from build123d import *

# Parameters (mm, degrees)
EXTRUDE1_DEPTH                         = 10
F_4_0_4_DIAMETER_HOLE1_D               = 3.9
F_4_0_4_DIAMETER_HOLE1_DEPTH           = 15
F_4_0_4_DIAMETER_HOLE1_ON_FACE_2_D     = 3.9
F_4_0_4_DIAMETER_HOLE1_ON_FACE_2_DEPTH = 15
SKETCH3_W                              = 10
SKETCH3_H                              = 8
EXTRUDE2_DEPTH                         = 10
F_4_0_4_DIAMETER_HOLE2_D               = 3.9
F_4_0_4_DIAMETER_HOLE2_DEPTH           = 15


with BuildPart() as part:
    # Sketch1 → Extrude1 (new body)
    with BuildSketch(Plane.XY):
        Polygon((-43.75, -15), (-43.75, -5), (23.75, 15), (43.75, 15), (43.75, -15), align=None)
    extrude(amount=EXTRUDE1_DEPTH)

    # Ø4.0 (4) Diameter Hole1
    with Locations(Plane(origin=(-43.75, -10, 5), x_dir=(0, 0, -1), z_dir=(-1, 0, 0))):
        with Locations((0, 0)):
            Hole(F_4_0_4_DIAMETER_HOLE1_D / 2, depth=F_4_0_4_DIAMETER_HOLE1_DEPTH)

    # Ø4.0 (4) Diameter Hole1 on face 2
    with Locations(Plane(origin=(43.75, -10, 5), x_dir=(0, 0, 1), z_dir=(1, 0, 0))):
        with Locations((0, 0), (0, -20)):
            Hole(F_4_0_4_DIAMETER_HOLE1_ON_FACE_2_D / 2, depth=F_4_0_4_DIAMETER_HOLE1_ON_FACE_2_DEPTH)

    # Sketch3 → Extrude2 (add)
    with BuildSketch(Plane.XY):
        with Locations((-38.75, -19)):
            Rectangle(SKETCH3_W, SKETCH3_H)
    extrude(amount=EXTRUDE2_DEPTH)

    # Ø4.0 (4) Diameter Hole2
    with Locations(Plane(origin=(-43.75, -18, 5), x_dir=(0, 0, -1), z_dir=(-1, 0, 0))):
        with Locations((0, 0)):
            Hole(F_4_0_4_DIAMETER_HOLE2_D / 2, depth=F_4_0_4_DIAMETER_HOLE2_DEPTH)


solid = part.part
Here's how the part is built. I have some questions about the finished solid (model axes, mm). A direction names the side the tool comes from. Coordinates: 2 decimals unless noted, no trailing zeros. Order: outer loops, then holes, each group sorted by start corner. A loop starts at its lowest first (then second) coordinate and runs counter-clockwise, first axis right, second up. Notation, with made-up numbers: M 58,-27 L 101,-27 A18 ccw 101,6 Z; hole C 57,81 d10. An arc over 180 degrees is marked long. Answer as CSV lines item,"result". Start each with the question number.
1. On a 3-axis mill with a long thin cutter (end or side, diameter ignored), from which of +Z, -Z, +X, -X, +Y, -Y can I reach the whole of each face in a straight line? I mean faces 4 (the cylindrical face through (36.145, 9.914, 6.948)), 5 (the flat face through (-33.75, -20, 4)), 6 (the flat face through (-28.75, -10, 5)). Say none if no direction works.
2. We'd pull the mould along Y, two halves only. Please class faces 1 (the cylindrical face through (-36.145, -8.813, 3.453)), 2 (the flat face through (9, -4, 0)), 3 (the flat face through (6, -15, 5)): released by +Y, released by -Y, zero draft, split by the parting line, or undercut.
3. I need wall thicknesses on line 1 (Y direction, x = 35, z = 5); line 2 (Z direction, x = -41.25, y = -18); line 3 (Y direction, x = -37.25, z = 5). Which ranges of each line are inside material? Lowest first, please. Write a range as [from, to].
4. I want a section at B-B, the plane z = 5. Write out the boundary of the cut face in (x, y).
5. I want a section at C-C, the plane y = -10. Write out the boundary of the cut face in (x, z), and give its area (3 significant figures).
6. I want a section at A-A, the plane y = -18. Write out the boundary of the cut face in (x, z).
7. For pin 1 (6 mm diameter, centred on x = 29, z = 6.5, fed in from -Y); pin 2 (1.2 mm diameter, centred on y = 9.5, z = 4.5, fed in from +X); pin 3 (6 mm diameter, centred on x = -4.5, z = 7.5, fed in from +Y); pin 4 (4 mm diameter, centred on x = -21.5, y = -14, fed in from -Z), each with a flat end and sliding along its axis, tell me the tip position at first contact or that it passes through.
8. I want a section at D-D, the plane x = 0. Write out the boundary of the cut face in (y, z).
Recorded:
1,face 4,"+X"
1,face 5,"+Z, -Z, +X, -Y"
1,face 6,"-X"
2,face 1,"undercut"
2,face 2,"zero draft"
2,face 3,"released by -Y"
3,line 1,"y = [-15, -11.95], [-8.05, 8.05], [11.95, 15]"
3,line 2,"z = [0, 3.05], [6.95, 10]"
3,line 3,"y = [-23, -19.95], [-16.05, -11.95], [-8.05, -3.07]"
4,outline,"M -43.75,-23 L -33.75,-23 L -33.75,-19.95 L -43.75,-19.95 Z; M -43.75,-16.05 L -33.75,-16.05 L -33.75,-15 L 43.75,-15 L 43.75,-11.95 L 28.75,-11.95 L 28.75,-8.05 L 43.75,-8.05 L 43.75,8.05 L 28.75,8.05 L 28.75,11.95 L 43.75,11.95 L 43.75,15 L 23.75,15 L -43.75,-5 L -43.75,-8.05 L -28.75,-8.05 L -28.75,-11.95 L -43.75,-11.95 Z"
5,outline,"M -43.75,0 L 43.75,0 L 43.75,3.05 L 28.75,3.05 L 28.75,6.95 L 43.75,6.95 L 43.75,10 L -43.75,10 L -43.75,6.95 L -28.75,6.95 L -28.75,3.05 L -43.75,3.05 Z"
5,area,"758 mm2"
6,outline,"M -43.75,0 L -33.75,0 L -33.75,3.05 L -43.75,3.05 Z; M -43.75,6.95 L -33.75,6.95 L -33.75,10 L -43.75,10 Z"
7,pin 1,"stops at y = -15"
7,pin 2,"stops at x = 28.75"
7,pin 3,"stops at y = 7.52"
7,pin 4,"stops at z = 0"
8,outline,"M -15,0 L 7.96,0 L 7.96,10 L -15,10 Z"
